Geometry: final body of the model. Coordinates: model frame, mm. A direction names the side the tool comes from. Give positions to 0.01 mm unless a question says otherwise; leave off trailing zeros. Write each loop counter-clockwise with the first axis right and the second up, starting at its lowest first coordinate (ties: lowest second). Pieces come first, ordered by that corner, then holes.
Q1. Section C-C (y = -7.5). Return the cut outline in (x, z).
Q2. Line query: line 1 (X direction, y = -8.5, z = 3.5); line 2 (Y direction, x = 59.5, z = 21); line 3 (Z direction, x = 29, y = -5). Output: solid intervals per line, ascending.
Q3. Section A-A (y = -33.5). Return the cut outline in (x, z).
Q4. Section D-D (x = 54). Return the cut outline in (y, z).
Q5. Mould query, pull axis X, two halves, no side actions, for faces 4 (the flat face through (11, -20, 11)), 5 (the flat face through (57.15, -19, 6)), 6 (the flat face through (9, -19, 0)). Classes: +X half, -X half, draft (parallel to the pull), parting line (faces both ways), or undercut.
Q6. Section B-B (z = 36). Return the cut outline in (x, y).
Q7. Pin query (flat end, axial travel): pin 1 Ø9 at (x, y) = (46.5, -17.5) entering from -Z; pin 2 Ø8 at (x, z) = (66, 22) entering from -Y; pin 3 Ø14 at (y, z) = (-27, 8) entering from -X. Return the tip coordinate at first contact, or that it passes through.
Q8. Reachability of faces 1 (the flat face through (61.7, -22.4, 14.5)), 2 (the flat face through (19.05, -19, 6)), 3 (the flat face through (29, -12.7, 31)) from +Z, -Z, +X, -X, +Y, -Y: full face, straight path, thin tool, end or side. Return the list, or none.
from build123d import *

# Parameters (mm, degrees)
F1_DEPTH = 12.7
F2_DEPTH = 38.1
F4_DEPTH = 76.2


with BuildPart() as f1:
    # F0 (on Front) → F1 (new body)
    with BuildSketch(Plane.XZ):
        Polygon((0, 25.4), (0, 0), (38.1, 38.1), (76.2, 0), (76.2, 25.4), (50.8, 50.8), (25.4, 50.8), align=None)
    extrude(amount=F1_DEPTH)

    # F0 (on Front) → F2 (join)
    with BuildSketch(Plane.XZ):
        Polygon((38.1, 38.1), (0, 0), (19.05, 0), (19.05, 12.7), (57.15, 12.7), (57.15, 0), (76.2, 0), align=None)
    extrude(amount=F2_DEPTH)

    # F3 (on Right) → F4 (cut)
    with BuildSketch(Plane.YZ):
        Polygon((-12.7, 38.1), (-38.1, 38.1), (-38.1, 0), align=None)
    extrude(amount=F4_DEPTH, mode=Mode.SUBTRACT)


solid = f1.part
Computed:
1. outline: (0, 0) - (19.05, 0) - (19.05, 12.7) - (57.15, 12.7) - (57.15, 0) - (76.2, 0) - (76.2, 25.4) - (50.8, 50.8) - (25.4, 50.8) - (0, 25.4) - close
2. line 1: x = 0 to 19.05, 57.15 to 76.2
2. line 2: y = -12.7 to 0
2. line 3: z = 12.7 to 50.8
3. outline: (0, 0) - (19.05, 0) - (19.05, 6.9) - (6.9, 6.9) - close; (57.15, 0) - (76.2, 0) - (69.3, 6.9) - (57.15, 6.9) - close
4. outline: (-29.63, 12.7) - (0, 12.7) - (0, 47.6) - (-12.7, 47.6) - (-12.7, 22.2) - (-23.3, 22.2) - close
5. face 4: -X half
5. face 5: undercut
5. face 6: draft
6. outline: (10.6, -12.7) - (36, -12.7) - (36, -14.1) - (40.2, -14.1) - (40.2, -12.7) - (65.6, -12.7) - (65.6, 0) - (10.6, 0) - close
7. pin 1: stops at z = 12.7
7. pin 2: stops at y = -12.7
7. pin 3: stops at x = 1
8. face 1: +Z, +X, -Y
8. face 2: -Z, +Y, -Y
8. face 3: +Z, -Y
